```python
from build123d import *

# Parameters (mm, degrees)
SALIENTE_EXTRUIR1_OUTLINE_R   = 0.901496021
SALIENTE_EXTRUIR1_OUTLINE_R_2 = 1.5
SALIENTE_EXTRUIR1_DEPTH       = 2.5
CROQUIS2_R                    = 3
SALIENTE_EXTRUIR2_DEPTH       = 5
REDONDEO1_R                   = 2.5


# Read off the part's stored shape, not the designer's step: Saliente-Extruir1
with BuildPart() as part:
    # Saliente-Extruir1 outline → Saliente-Extruir1 (new body)
    with BuildSketch(Plane.XY.offset(-107.5)):
        with BuildLine():
            ThreePointArc((173.644297207, -49.239284265), (177.488489802, -47.444240173), (175.69344571, -43.600047578))
            Line((175.69344571, -43.600047578), (154.076371743, -35.744978316))
            ThreePointArc((154.076371743, -35.744978316), (150.794254841, -36.588868647), (150.392873293, -39.953885006))
            Line((150.392873293, -39.953885006), (152.021065929, -41.381969984))
            ThreePointArc((152.021065929, -41.381969984), (152.024143972, -41.383094175), (152.02722324, -41.384215004))
            Line((152.02722324, -41.384215004), (173.644297207, -49.239284265))
        make_face()
        with Locations((174.668871458, -46.419665921)):
            Circle(SALIENTE_EXTRUIR1_OUTLINE_R, mode=Mode.SUBTRACT)
        with Locations((153.051797492, -38.564596659)):
            Circle(SALIENTE_EXTRUIR1_OUTLINE_R_2, mode=Mode.SUBTRACT)
    extrude(amount=SALIENTE_EXTRUIR1_DEPTH)

    # Croquis2 → Saliente-Extruir2 (add)
    with BuildSketch(Plane.XY.offset(-105)):
        with Locations(Location((174.668871458, -46.419665921, 0), (0, 0, 250.030202639))):
            Circle(CROQUIS2_R)
    extrude(amount=SALIENTE_EXTRUIR2_DEPTH)

    # Redondeo1
    redondeo1_edges = [part.edges().sort_by_distance(p)[0] for p in [
        (175.69344571, -43.600047578, -100),
    ]]
    fillet(redondeo1_edges, radius=REDONDEO1_R)


solid = part.part
```
Geometry: final body of the model. Coordinates: model frame, mm. A direction names the side the tool comes from. Round coordinates to 2 decimals unless told otherwise and drop trailing zeros. Order: outer loops, then holes, each group sorted by start corner. A loop starts at its lowest first (then second) coordinate and runs counter-clockwise, first axis right, second up. Notation, with made-up numbers: (-37, -2.75) -> (19, -2.75) arc R20 cw to (19, 8.25) -> close; hole circle Ø11 at (-11, -14.75). An arc over 180 degrees is marked (long way). Use one line per item in the form item = value. Start each with the question number.
1. Draft query along Y for faces 1 (the face through (175, -46, -105)), 2 (the face through (151.2, -40.66, -106.27)), 3 (the face through (165.04, -39.73, -106.27)). Return one class per face: pulls with the +Y half, pulls with the -Y half, needs draft (parallel to the pull), parting line crosses it, or undercut.
2. Line query: probe 1 along Z at (x, y) = (171, -46.75); probe 2 along Y at (x, z) = (152.5, -107); probe 3 along X at (y, z) = (-45.5, -102.75). Output: solid intervals per line, ascending.
3. Cut plane D-D (y = -36.5). Return the cut outline in (x, z).
4. Pin query (flat end, axial travel): pin 1 Ø5 at (x, y) = (158, -46.5) entering from -Z; pin 2 Ø1.5 at (y, z) = (-45, -102.5) entering from +X; pin 3 Ø1.5 at (x, z) = (172.5, -104) entering from +Y; pin 4 Ø4 at (x, y) = (168, -44.5) entering from +Z. Return the tip coordinate at first contact, or that it passes through.
5. Cut plane A-A (y = -38). Return the cut outline in (x, z), then the cut area to 3 significant figures.
6. Reachability of faces 4 (the face through (151.553, -38.499, -106.268)), 5 (the face through (173.77, -46.38, -106.27)) from +Z, -Z, +X, -X, +Y, -Y: full face, straight path, thin tool, end or side. Return the list, or none.
7. Cut plane B-B (z = -105.5). Count the separate pieces of the cut face and the enclosed holes in it, then the cut area to 3 significant figures.
8. Cut plane C-C (x = 168.25). Return the cut outline in (y, z).
Solution:
q1.face_1 = undercut
q1.face_2 = pulls with the -Y half
q1.face_3 = pulls with the +Y half
q2.probe_1 = -107.5 to -105
q2.probe_2 = -41.56 to -39.96, -37.17 to -35.62
q2.probe_3 = 171.81 to 177.52
q3.outline = (150.88, -107.5) -> (156.15, -107.5) -> (156.15, -105) -> (150.88, -105) -> close
q4.pin_1 = through
q4.pin_2 = 177.59
q4.pin_3 = -43.78
q4.pin_4 = -105
q5.outline = (150.11, -107.5) -> (151.66, -107.5) -> (151.66, -105) -> (150.11, -105) -> close; (154.44, -107.5) -> (160.28, -107.5) -> (160.28, -105) -> (154.44, -105) -> close
q5.area = 18.5 mm^2
q6.face_4 = +Z, -Z
q6.face_5 = -Z
q7.separate_pieces = 1
q7.enclosed_holes = 2
q7.area = 156 mm^2
q8.outline = (-47.28, -107.5) -> (-40.9, -107.5) -> (-40.9, -105) -> (-47.28, -105) -> close
